```python
from build123d import *

# Parameters (mm, degrees)
SKETCH_1_R          = 9.75
EXTRUDE_1_DEPTH     = 140
SKETCH_2_W          = 34
SKETCH_2_H          = 24
EXTRUDE_2_DEPTH     = 50
CUT_EXTRUDE_1_REACH = 143.722


with BuildPart() as part:
    # 스케치1 → 보스-돌출1 (new body)
    with BuildSketch(Plane.XY):
        Circle(SKETCH_1_R)
    extrude(amount=EXTRUDE_1_DEPTH)

    # 스케치2 → 보스-돌출2 (add)
    with BuildSketch(Plane.XY):
        with Locations((0, 2)):
            Rectangle(SKETCH_2_W, SKETCH_2_H)
    extrude(amount=-EXTRUDE_2_DEPTH)

    # 스케치3 → 컷-돌출1 (cut, up to next)
    with BuildSketch(Plane.XY, mode=Mode.PRIVATE) as cut_extrude_1_sk1:
        with BuildLine():
            Line((-6.519202405, -7.25), (-17, -7.25))
            Line((-17, -7.25), (-17, -10))
            Line((-17, -10), (17, -10))
            Line((17, -10), (17, -7.25))
            Line((17, -7.25), (6.519202405, -7.25))
            ThreePointArc((6.519202405, -7.25), (0, -9.75), (-6.519202405, -7.25))
        make_face()
    cut_extrude_1_tool1 = extrude(cut_extrude_1_sk1.sketch, amount=-CUT_EXTRUDE_1_REACH, mode=Mode.PRIVATE) & part.part
    add(cut_extrude_1_tool1.solids().sort_by_distance((0, -9.784111, 0))[0], mode=Mode.SUBTRACT)


solid = part.part
```
The model under review builds one solid part; all positions refer to its coordinate system, in mm. A direction names the side the tool comes from. Round coordinates to 2 decimals unless told otherwise and drop trailing zeros. Loops run counter-clockwise (first coordinate to the right, second up) from the corner with the lowest first, then second, coordinate; pieces in that order, holes last. Notation, with made-up numbers: (70.25, -1.75) -> (74.25, -1.75) arc R8 ccw to (74.25, 10.25) -> close; hole circle Ø8 at (63.25, -23). An arc over 180 degrees is marked (long way). Answer as a JSON object with one key per item and string values. Group by question number.
1) For line 1 (Z direction, x = -13.5, y = 1.75); line 2 (X direction, y = -7.25, z = 100.5); line 3 (Y direction, x = 0, z = -11.5), list the stretches that pass through material, from the lowest coordinate up. Write a range as [from, to].
2) We need section C-C on z = 72. Write out the cut boundary in (x, y).
3) For pin 1 Ø4 at (x, z) = (-10, 18) entering from -Y; pin 2 Ø6 at (y, z) = (1, 96.5) entering from -X; pin 3 Ø5 at (x, z) = (9.5, -13) entering from -Y, all flat-tipped, find the tip position at first contact; note any pin that passes through.
4) For faces 1 (the face through (-12, -7.25, -25)), 2 (the face through (0, 14, -25)), 3 (the face through (12, -7.25, -25)), list the 3-axis set-ups (+Z, -Z, +X, -X, +Y, -Y) from which the entire face can be reached by the end or side of a thin tool; tool diameter is ignored.
5) We need section D-D on y = 12.25. Write out the cut boundary in (x, z), then the cut area to 3 significant figures.
6) We need section A-A on y = 4.5. Write out the cut boundary in (x, z), then the cut area to 3 significant figures.
7) We need section B-B on x = 0. Write out the cut boundary in (y, z).
Result set:
{
 "1": {"line 1": "[-50, 0]", "line 2": "[-6.52, 6.52]", "line 3": "[-9.75, 14]"},
 "2": {"outline": "circle Ø19.5 at (0, 0)"},
 "3": {"pin 1": "y = -5.57", "pin 2": "x = -9.75", "pin 3": "y = -7.25"},
 "4": {"face 1": "+Z, -Z, -X, -Y", "face 2": "+Z, -Z, +X, -X, +Y", "face 3": "+Z, -Z, +X, -Y"},
 "5": {"outline": "(-17, -50) -> (17, -50) -> (17, 0) -> (-17, 0) -> close", "area": "1,700 mm²"},
 "6": {"outline": "(-17, -50) -> (17, -50) -> (17, 0) -> (8.65, 0) -> (8.65, 140) -> (-8.65, 140) -> (-8.65, 0) -> (-17, 0) -> close", "area": "4,120 mm²"},
 "7": {"outline": "(-9.75, -50) -> (14, -50) -> (14, 0) -> (9.75, 0) -> (9.75, 140) -> (-9.75, 140) -> close"}
}
